```python
from build123d import *

# Parameters (mm, degrees)
SKETCH1_W           = 20
SKETCH1_H           = 5
BOSS_EXTRUDE1_DEPTH = 10
CUT_EXTRUDE1_DEPTH  = 16
SKETCH8_R           = 0.915
CUT_EXTRUDE6_DEPTH  = 23.5
SKETCH7_R           = 0.915
CUT_EXTRUDE5_DEPTH  = 23.5
SKETCH10_R          = 2.5
BOSS_EXTRUDE4_DEPTH = 1
SKETCH5_W           = 10
SKETCH5_H           = 8.4
BOSS_EXTRUDE3_DEPTH = 5
SKETCH6_R           = 1
CUT_EXTRUDE4_DEPTH  = 16
CUT_EXTRUDE7_REACH  = 20.364
SKETCH9_R           = 0.915
SKETCH11_R          = 0.975
CUT_EXTRUDE8_DEPTH  = 16.362291535
CHAMFER1_SIZE       = 1
FILLET1_R           = 1


with BuildPart() as part:
    # Sketch1 → Boss-Extrude1 (new body)
    with BuildSketch(Plane(origin=(0, 0, 0), x_dir=(1, 0, 0), z_dir=(0, 1, 0))):
        Rectangle(SKETCH1_W, SKETCH1_H)
    extrude(amount=BOSS_EXTRUDE1_DEPTH)

    # Sketch2 → Cut-Extrude1 (cut, through all)
    with BuildSketch(Plane.XY.offset(2.5)):
        Polygon((3.714359354, 10), (-3.714359354, 10), (-5.1, 7.6), (5.1, 7.6), align=None)
    extrude(amount=-CUT_EXTRUDE1_DEPTH, mode=Mode.SUBTRACT)

    # Sketch8 → Cut-Extrude6 (cut, through all)
    with BuildSketch(Plane(origin=(10, 0, 0), x_dir=(0, 0, -1), z_dir=(1, 0, 0))):
        with Locations((0, 7.6)):
            Circle(SKETCH8_R)
    extrude(amount=-CUT_EXTRUDE6_DEPTH, mode=Mode.SUBTRACT)

    # Sketch7 → Cut-Extrude5 (cut, through all)
    with BuildSketch(Plane(origin=(10, 0, 0), x_dir=(0, 0, -1), z_dir=(1, 0, 0))):
        with Locations((0, 2.6)):
            Circle(SKETCH7_R)
    extrude(amount=-CUT_EXTRUDE5_DEPTH, mode=Mode.SUBTRACT)

    # Sketch10 → Boss-Extrude4 (add)
    with BuildSketch(Plane.XY.offset(2.5)):
        with Locations(Location((0, 2.6, 0), (0, 0, 180))):
            Circle(SKETCH10_R)
    extrude(amount=BOSS_EXTRUDE4_DEPTH)

    # Sketch5 → Boss-Extrude3 (add)
    with BuildSketch(Plane(origin=(0, 0, -2.5), x_dir=(-1, 0, 0), z_dir=(0, 0, -1))):
        with Locations((0, -4.2)):
            Rectangle(SKETCH5_W, SKETCH5_H)
    extrude(amount=-BOSS_EXTRUDE3_DEPTH)

    # Sketch6 → Cut-Extrude4 (cut, through all)
    with BuildSketch(Plane.XY.offset(2.5)):
        with Locations((0, -4.4)):
            Circle(SKETCH6_R)
    extrude(amount=-CUT_EXTRUDE4_DEPTH, mode=Mode.SUBTRACT)

    # Cut-Extrude7: up to this face of the body (flat: up to its plane)
    cut_extrude7_end = Plane(part.part.faces().sort_by_distance((-5, -4.2, 0))[0])
    # Sketch9 → Cut-Extrude7 (cut, up to the picked face)
    with BuildSketch(Plane(origin=(5, 0, 0), x_dir=(0, 0, -1), z_dir=(1, 0, 0)), mode=Mode.PRIVATE) as cut_extrude7_sk1:
        with Locations((0, -4.4)):
            Circle(SKETCH9_R)
    cut_extrude7_tool1 = split(extrude(cut_extrude7_sk1.sketch, amount=-CUT_EXTRUDE7_REACH, mode=Mode.PRIVATE), bisect_by=cut_extrude7_end, keep=Keep.BOTH, mode=Mode.PRIVATE)
    add(cut_extrude7_tool1.solids().sort_by(Axis((5, -4.4, 0), (-1, 0, 0)))[0], mode=Mode.SUBTRACT)

    # Sketch11 → Cut-Extrude8 (cut, through all)
    with BuildSketch(Plane.XY.offset(3.5)):
        with Locations((0, 2.6)):
            Circle(SKETCH11_R)
    extrude(amount=-CUT_EXTRUDE8_DEPTH, mode=Mode.SUBTRACT)

    # Chamfer1
    chamfer1_edges = [part.edges().sort_by_distance(p)[0] for p in [
        (2.5, 2.6, 2.5),
    ]]
    chamfer(chamfer1_edges, length=CHAMFER1_SIZE - 0.0001)  # a hair under: the kernel refuses the full size

    # Fillet1
    fillet1_edges = [part.edges().sort_by_distance(p)[0] for p in [
        (-10, 0, 0),
        (-5, -8.4, 0),
        (5, -8.4, 0),
        (10, 0, 0),
    ]]
    fillet(fillet1_edges, radius=FILLET1_R)


solid = part.part
```
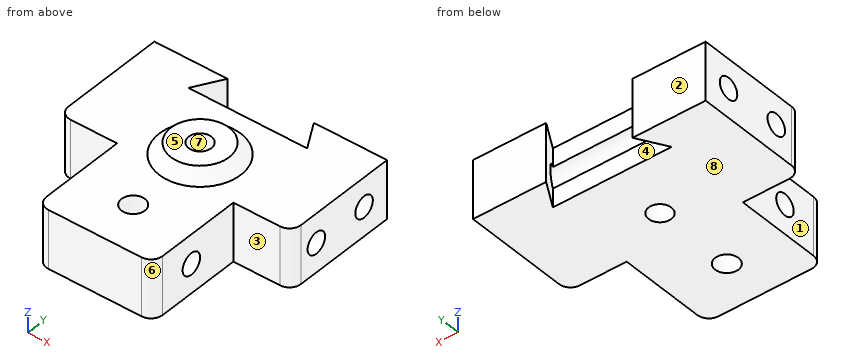
Read the model definition and answer for the solid it produces. Units are mm, in the model's axes. Face numbers are marked on the shaded views. A direction names the side the tool comes from. Coordinates: 2 decimals unless noted, no trailing zeros. Write each loop counter-clockwise with the first axis right and the second up, starting at its lowest first coordinate (ties: lowest second). Pieces come first, ordered by that corner, then holes. Notation, with made-up numbers: (24, 34.5) -> (34, 34.5) arc R23 ccw to (34, 49.5) -> close; hole circle Ø8 at (46, -9). An arc over 180 degrees is marked (long way). Write item = value, one per line.
(1) Section C-C on z = 1.5 is taken. Write down the section's boundary in (x, y) (3 decimals), plus the area to 3 significant figures.
From the geometry:
outline = (-10, 1) arc R1 ccw to (-9, 0) -> (-5, 0) -> (-5, -7.4) arc R1 ccw to (-4, -8.4) -> (4, -8.4) arc R1 ccw to (5, -7.4) -> (5, 0) -> (9, 0) arc R1 ccw to (10, 1) -> (10, 10) -> (3.714, 10) -> (5.1, 7.6) -> (-5.1, 7.6) -> (-3.714, 10) -> (-10, 10) -> close; hole circle Ø2 at (0, -4.4); hole circle Ø1.95 at (0, 2.6)
area = 256 mm2
(2) Section A-A on y = -4.4 is taken. Write down the section's boundary in (x, z) (3 decimals), plus the area to 3 significant figures.
From the geometry:
outline = (-5, -2.5) -> (-1, -2.5) -> (-1, -0.915) -> (-5, -0.915) -> close; (-5, 0.915) -> (-1, 0.915) -> (-1, 2.5) -> (-5, 2.5) -> close; (1, -2.5) -> (5, -2.5) -> (5, -0.915) -> (1, -0.915) -> close; (1, 0.915) -> (5, 0.915) -> (5, 2.5) -> (1, 2.5) -> close
area = 25.4 mm2
(3) Section D-D on x = -6.25 is taken. Write down the section's boundary in (y, z) (3 decimals), plus the area to 3 significant figures.
From the geometry:
outline = (0, -2.5) -> (10, -2.5) -> (10, 2.5) -> (0, 2.5) -> close; hole circle Ø1.83 at (2.6, 0); hole circle Ø1.83 at (7.6, 0)
area = 44.7 mm2
(4) Straight lines are drawn through the part: L1, parallel to Y at x = 0.5, z = 0 (3 decimals); L2, parallel to Y at x = -6.5, z = 0 (3 decimals); L3, parallel to X at y = 2.6, z = 1.5 (3 decimals). For each, find the intervals that lie inside material, in ascending order. Write a range as from..to.
From the geometry:
L1 = -8.4..-5.315, -3.485..1.685, 3.515..6.685
L2 = 0..1.685, 3.515..6.685, 8.515..10
L3 = -10..-0.975, 0.975..10
(5) For a pull along X with two mould halves and no side action, classify the marked faces 6, 7 and 8 as +X half, -X half, draft (parallel to the pull), parting line (faces both ways), or undercut.
From the geometry:
face_6 = +X half
face_7 = undercut
face_8 = draft
(6) Section B-B on x = 0 is taken. Count the separate pieces of the cut face and the enclosed holes in it, plus the area to 3 significant figures.
From the geometry:
separate_pieces = 3
enclosed_holes = 0
area = 63.0 mm2
(7) Given pin 1 Ø6 at (x, y) = (-4, -5) entering from +Z; pin 2 Ø3 at (y, z) = (2.6, 0) entering from +X; pin 3 Ø1.8 at (x, y) = (0, 2.6) entering from +Z; pin 4 Ø2.5 at (y, z) = (-5, 0.5) entering from -X, each flat-ended and moving along its own axis, determine where each tip first touches the part or whether it passes through.
From the geometry:
pin_1 = 2.5
pin_2 = 10
pin_3 = through
pin_4 = -5
(8) Which of the six approach directions +Z, -Z, +X, -X, +Y, -Y give full straight-line access (tool end or side, diameter ignored) to the marked faces 1, 2, 3, 4 and 5?
From the geometry:
face_1 = +Z, -Z, -X, -Y
face_2 = +Z, -Z, +X, -X, +Y
face_3 = +Z, -Z, +X, -Y
face_4 = +Z, -Z
face_5 = +Z, +X, -X, +Y, -Y
